Geometry: final body of the model. Coordinates: model frame, mm. Face numbers are marked on the shaded views. A direction names the side the tool comes from. Give positions to 0.01 mm unless a question says otherwise; leave off trailing zeros. Write each loop counter-clockwise with the first axis right and the second up, starting at its lowest first coordinate (ties: lowest second). Pieces come first, ordered by that corner, then holes.
Q1. Cut plane A-A on y = 3. Return the cut outline in (x, z).
Q2. Reachability of the marked faces 1 and 2 from +Z, -Z, +X, -X, +Y, -Y: full face, straight path, thin tool, end or side. Return the list, or none.
Q3. Cut plane C-C on y = 9. Return the cut outline in (x, z), plus the area to 3 significant figures.
Q4. Pin query (flat end, axial travel): pin 1 (4 mm diameter, centred on x = -112.75, z = 0, fed in from -Y); pin 2 (1.5 mm diameter, centred on y = 5.5, z = 16.5, fed in from +X); pin 3 (2 mm diameter, centred on y = 1.5, z = -16, fed in from +X). Return the tip coordinate at first contact, or that it passes through.
Q5. Draft query along X for the marked faces 3, 4, 5 and 6. Return one class per face: pulls with the +X half, pulls with the -X half, needs draft (parallel to the pull), parting line crosses it, or undercut.
Q6. Cut plane B-B on z = 0. Count the separate pieces of the cut face and the enclosed holes in it, plus the area to 3 significant figures.
Q7. Line query: L1, parallel to X at y = 13.75, z = 3; L2, parallel to X at y = 9.75, z = 6; L3, parallel to Y at x = -135, z = 6.5. Output: solid intervals per line, ascending.
```python
from build123d import *

# Parameters (mm, degrees)
SALIENTE_EXTRUIR7_DEPTH = 14
CROQUIS4_R              = 18
CORTAR_EXTRUIR1_DEPTH   = 7
CROQUIS5_R              = 3.75
CROQUIS5_R_2            = 1.5
CROQUIS5_R_3            = 1.702426791
CORTAR_EXTRUIR3_DEPTH   = 144.864519601
CROQUIS6_R              = 3.75
CROQUIS6_R_2            = 1.5
CORTAR_EXTRUIR4_DEPTH   = 144.864519601
REDONDEO2_R             = 1


with BuildPart() as part:
    # Croquis1 → Saliente-Extruir7 (new body)
    with BuildSketch(Plane(origin=(0, 0, 0), x_dir=(1, 0, 0), z_dir=(0, 1, 0))):
        with BuildLine():
            ThreePointArc((-120, 22), (-142, 0), (-120, -22))
            ThreePointArc((-120, -22), (-60.008802525, -15.348556021), (0, -21.839249444))
            ThreePointArc((0, -21.839249444), (21.839249444, 0), (0, 21.839249444))
            ThreePointArc((0, 21.839249444), (-60.008802533, 15.348549982), (-120, 22))
        make_face()
    extrude(amount=SALIENTE_EXTRUIR7_DEPTH)

    # Croquis4 → Cortar-Extruir1 (cut)
    with BuildSketch(Plane(origin=(0, 14, 0), x_dir=(1, 0, 0), z_dir=(0, 1, 0))):
        with Locations(Location((-120, 0, 0), (0, 0, 270))):
            Circle(CROQUIS4_R)
        with Locations(Location((0, 0, 0), (0, 0, 270))):
            Circle(CROQUIS4_R)
    extrude(amount=-CORTAR_EXTRUIR1_DEPTH, mode=Mode.SUBTRACT)

    # Croquis5 → Cortar-Extruir3 (cut, through all)
    with BuildSketch(Plane(origin=(0, 7, 0), x_dir=(1, 0, 0), z_dir=(0, 1, 0))):
        with Locations(Location((-120, 0, 0), (0, 0, 270))):
            Circle(CROQUIS5_R)
        with Locations(Location((-127.25, 0, 0), (0, 0, 270))):
            Circle(CROQUIS5_R_2)
        with Locations(Location((-112.75, 0, 0), (0, 0, 270))):
            Circle(CROQUIS5_R_3)
    extrude(amount=-CORTAR_EXTRUIR3_DEPTH, mode=Mode.SUBTRACT)

    # Croquis6 → Cortar-Extruir4 (cut, through all)
    with BuildSketch(Plane(origin=(0, 7, 0), x_dir=(1, 0, 0), z_dir=(0, 1, 0))):
        with Locations(Location((0, 0, 0), (0, 0, 270))):
            Circle(CROQUIS6_R)
        with Locations(Location((7.25, 0, 0), (0, 0, 270))):
            Circle(CROQUIS6_R_2)
        with Locations(Location((-7.25, 0, 0), (0, 0, 270))):
            Circle(CROQUIS6_R_2)
    extrude(amount=-CORTAR_EXTRUIR4_DEPTH, mode=Mode.SUBTRACT)

    # Redondeo2
    # the kernel refuses this fillet: 1 mm, written as the material it takes off along each edge
    with BuildSketch(Plane(origin=(-59.637450549, 14, 292.562134942), x_dir=(-0.226540467768197, 0, -0.9740017538297179), z_dir=(-0.9740017538297179, 0, 0.226540467768197))) as redondeo2_piece_1:
        with BuildLine():
            CenterArc((277.21382765 + REDONDEO2_R, REDONDEO2_R), REDONDEO2_R, 180, 90)
            Line((277.21382765 + REDONDEO2_R, 0), (277.21382765, 0))
            Line((277.21382765, 0), (277.21382765, REDONDEO2_R))
        make_face()
    revolve(axis=Axis((-59.637450549, 14, 292.562134942), (0, -1, 0)), revolution_arc=26.03345413, mode=Mode.SUBTRACT)
    with BuildSketch(Plane(origin=(-120, 14, 0), x_dir=(0, 0, 1), z_dir=(-1, 0, 0))) as redondeo2_piece_2:
        with BuildLine():
            CenterArc((18 + REDONDEO2_R, -REDONDEO2_R), REDONDEO2_R, 90, 90)
            Line((18, -REDONDEO2_R), (18, 0))
            Line((18, 0), (18 + REDONDEO2_R, 0))
        make_face()
    revolve(axis=Axis((-120, 14, 0), (0, 1, 0)), mode=Mode.SUBTRACT)
    with BuildSketch(Plane(origin=(0, 14, 0), x_dir=(-0.11440584030720254, 0, 0.993434096306143), z_dir=(-0.993434096306143, 0, -0.11440584030720254))) as redondeo2_piece_3:
        with BuildLine():
            CenterArc((21.839249444 - REDONDEO2_R, -REDONDEO2_R), REDONDEO2_R, 0, 90)
            Line((21.839249444 - REDONDEO2_R, 0), (21.839249444, 0))
            Line((21.839249444, 0), (21.839249444, -REDONDEO2_R))
        make_face()
    revolve(axis=Axis((0, 14, 0), (0, 1, 0)), revolution_arc=193.138712049, mode=Mode.SUBTRACT)
    with BuildSketch(Plane(origin=(0, 14, 0), x_dir=(0, 0, 1), z_dir=(-1, 0, 0))) as redondeo2_piece_4:
        with BuildLine():
            CenterArc((18 + REDONDEO2_R, -REDONDEO2_R), REDONDEO2_R, 90, 90)
            Line((18, -REDONDEO2_R), (18, 0))
            Line((18, 0), (18 + REDONDEO2_R, 0))
        make_face()
    revolve(axis=Axis((0, 14, 0), (0, 1, 0)), mode=Mode.SUBTRACT)
    with BuildSketch(Plane(origin=(-59.637450891, 14, -292.561880174), x_dir=(0.22393033908793564, 0, 0.9746051524776391), z_dir=(0.9746051524776391, 0, -0.22393033908793564))) as redondeo2_piece_5:
        with BuildLine():
            CenterArc((277.213578921 + REDONDEO2_R, REDONDEO2_R), REDONDEO2_R, 180, 90)
            Line((277.213578921 + REDONDEO2_R, 0), (277.213578921, 0))
            Line((277.213578921, 0), (277.213578921, REDONDEO2_R))
        make_face()
    revolve(axis=Axis((-59.637450891, 14, -292.561880174), (0, -1, 0)), revolution_arc=26.033477851, mode=Mode.SUBTRACT)
    with BuildSketch(Plane(origin=(-120, 14, 0), x_dir=(0.11357352107267756, 0, -0.9935295945824433), z_dir=(0.9935295945824433, 0, 0.11357352107267756))) as redondeo2_piece_6:
        with BuildLine():
            CenterArc((22 - REDONDEO2_R, -REDONDEO2_R), REDONDEO2_R, 0, 90)
            Line((22, -REDONDEO2_R), (22, 0))
            Line((22, 0), (22 - REDONDEO2_R, 0))
        make_face()
    revolve(axis=Axis((-120, 14, 0), (0, 1, 0)), revolution_arc=193.042709536, mode=Mode.SUBTRACT)


solid = part.part
```
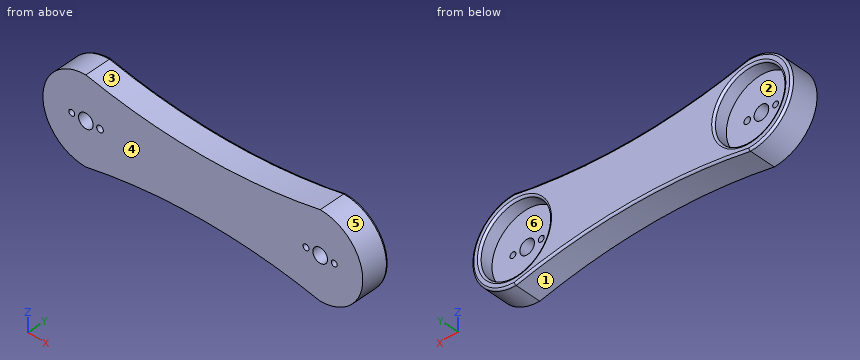
Data:
1. outline: (-120, -22) arc R277.21 cw to (0, -21.84) arc R21.84 ccw to (0, 21.84) arc R277.21 cw to (-120, 22) arc R22 ccw to start; hole circle Ø3 at (-127.25, 0); hole circle Ø7.5 at (-120, 0); hole circle Ø3.4 at (-112.75, 0); hole circle Ø3 at (-7.25, 0); hole circle Ø7.5 at (0, 0); hole circle Ø3 at (7.25, 0)
2. face 1: -Z, +Y, -Y
2. face 2: +Y
3. outline: (-120, -22) arc R277.21 cw to (0, -21.84) arc R21.84 ccw to (0, 21.84) arc R277.21 cw to (-120, 22) arc R22 ccw to start; hole circle Ø36 at (-120, 0); hole circle Ø36 at (0, 0)
3. area: 3,680 mm2
4. pin 1: stops at y = 0
4. pin 2: stops at x = 15.13
4. pin 3: stops at x = 15.87
5. face 3: undercut
5. face 4: needs draft
5. face 5: pulls with the +X half
5. face 6: undercut
6. separate pieces: 7
6. enclosed holes: 0
6. area: 1,600 mm2
7. L1: x = -141.45 to -138.09, -101.91 to -18.09, 18.09 to 21.29
7. L2: x = -141.17 to -136.97, -103.03 to -16.97, 16.97 to 21
7. L3: y = 0 to 7
